The figure shows three views and two pictorial views of one solid part (mm, origin at its lowest corner). Answer the questions. A direction names the side the tool comes from. Coordinates: 2 decimals unless noted, no trailing zeros. Order: outer loops, then holes, each group sorted by start corner. A loop starts at its lowest first (then second) coordinate and runs counter-clockwise, first axis right, second up. Notation, with made-up numbers: M -9,12.5 L 16,12.5 A20 cw 16,17.5 Z; hole C 59,-27 d2. An arc over 180 degrees is marked long. Answer in a Markdown table with one row per item. Add a question column.
Item 1: The part is cut by section C-C (x = 8). Write down the section's boundary in (y, z).
Item 2: The part is cut by section D-D (y = 75). Write down the section's boundary in (x, z).
Item 3: A flat-ended cylindrical pin translates along its axis: pin 1 Ø0.9 at (x, z) = (102, 1) entering from -Y. Find the tip coordinate at first contact, or state that the pin passes through.
Item 4: Which of the six approach directions +Z, -Z, +X, -X, +Y, -Y give full straight-line access (tool end or side, diameter ignored) to the marked faces 1 and 2?
Item 5: The part is cut by section A-A (y = 115). Write down the section's boundary in (x, z).
Item 6: The part is cut by section B-B (z = 11.25). Write down the section's boundary in (x, y), then the cut area to 3 significant figures.
Item 7: Consider line 1 (X direction, y = 75, z = 10.5); line 2 (Y direction, x = 8, z = 3.75); line 3 (X direction, y = 72, z = 7.75). Determine where each line is inside the solid, lowest interval first. Write a range as from..to.
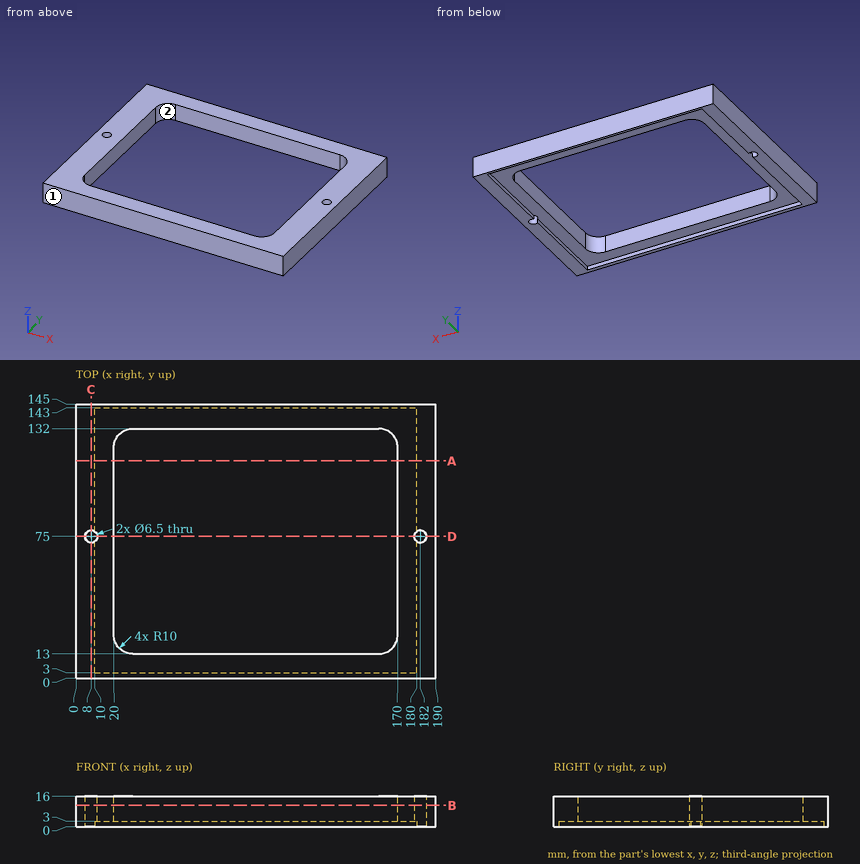
Reply:
| question | item | result |
|---|---|---|
| 1 | outline | M 0,0 L 71.75,0 L 71.75,16 L 0,16 Z; M 78.25,0 L 145,0 L 145,16 L 78.25,16 Z |
| 2 | outline | M 0,0 L 4.75,0 L 4.75,16 L 0,16 Z; M 11.25,3 L 20,3 L 20,16 L 11.25,16 Z; M 170,3 L 178.75,3 L 178.75,16 L 170,16 Z; M 185.25,0 L 190,0 L 190,16 L 185.25,16 Z |
| 3 | pin 1 | stops at y = 0 |
| 4 | face 1 | +Z, -Z, +X, -X, -Y |
| 4 | face 2 | +Z, -Z |
| 5 | outline | M 0,0 L 10,0 L 10,3 L 20,3 L 20,16 L 0,16 Z; M 170,3 L 180,3 L 180,0 L 190,0 L 190,16 L 170,16 Z |
| 6 | outline | M 0,0 L 190,0 L 190,145 L 0,145 Z; hole C 8,75 d6.5; hole M 20,23 A10 ccw 30,13 L 160,13 A10 ccw 170,23 L 170,122 A10 ccw 160,132 L 30,132 A10 ccw 20,122 Z; hole C 182,75 d6.5 |
| 6 | area | 9,720 mm2 |
| 7 | line 1 | x = 0..4.75, 11.25..20, 170..178.75, 185.25..190 |
| 7 | line 2 | y = 0..71.75, 78.25..145 |
| 7 | line 3 | x = 0..6.75, 9.25..20, 170..180.75, 183.25..190 |
